Verification items for the finished model (mm, model axes). A direction names the side the tool comes from. Round coordinates to 2 decimals unless told otherwise and drop trailing zeros. Order: outer loops, then holes, each group sorted by start corner. A loop starts at its lowest first (then second) coordinate and runs counter-clockwise, first axis right, second up. Notation, with made-up numbers: (21.5, 54.25) -> (40.5, 54.25) arc R16 ccw to (40.5, 77.25) -> close; hole circle Ø3 at (6.5, 11.5). An arc over 180 degrees is marked (long way). Write item = value, one per line. Start each with the question number.
from build123d import *

# Parameters (mm, degrees)
SKETCH_1_W      = 80
SKETCH_1_H      = 59.5
EXTRUDE_1_DEPTH = 5
FILLET_1_R      = 1
EXTRUDE_2_DEPTH = 1
CHAMFER_1_SIZE  = 0.8
EXTRUDE_START   = -1
EXTRUDE_3_DEPTH = 1
CHAMFER_2_SIZE  = 0.8


with BuildPart() as part:
    # 草图1 → 凸台-拉伸1 (new body)
    with BuildSketch(Plane(origin=(0, 0, 0), x_dir=(1, 0, 0), z_dir=(0, 1, 0))):
        with Locations((59.287159713, -12.081031523)):
            Rectangle(SKETCH_1_W, SKETCH_1_H)
    extrude(amount=EXTRUDE_1_DEPTH)

    # 圆角1
    fillet_1_edges = [part.edges().sort_by_distance(p)[0] for p in [
        (59.287159713, 5, -17.668968477),
        (59.287159713, 0, -17.668968477),
        (59.287159713, 0, 41.831031523),
        (59.287159713, 5, 41.831031523),
    ]]
    fillet(fillet_1_edges, radius=FILLET_1_R)

    # 草图2 → 凸台-拉伸2 (add)
    with BuildSketch(Plane(origin=(99.287159713, 0, 0), x_dir=(0, 0, -1), z_dir=(1, 0, 0))):
        with BuildLine():
            Line((16.668968477, 5.5), (-40.831031523, 5.5))
            ThreePointArc((-40.831031523, 5.5), (-41.891691695, 5.060660172), (-42.331031523, 4))
            Line((-42.331031523, 4), (-42.331031523, 1))
            ThreePointArc((-42.331031523, 1), (-41.891691695, -0.060660172), (-40.831031523, -0.5))
            Line((-40.831031523, -0.5), (16.668968477, -0.5))
            ThreePointArc((16.668968477, -0.5), (17.729628648, -0.060660172), (18.168968477, 1))
            Line((18.168968477, 1), (18.168968477, 4))
            ThreePointArc((18.168968477, 4), (17.729628648, 5.060660172), (16.668968477, 5.5))
        make_face()
    extrude(amount=-EXTRUDE_2_DEPTH)

    # 倒角1
    chamfer_1_edges = [part.edges().sort_by_distance(p)[0] for p in [
        (99.287159713, 5.060660172, -17.729628648),
        (99.287159713, 5.5, 12.081031523),
        (99.287159713, 5.060660172, 41.891691695),
        (99.287159713, 2.5, 42.331031523),
        (99.287159713, -0.060660172, 41.891691695),
        (99.287159713, -0.5, 12.081031523),
        (99.287159713, -0.060660172, -17.729628648),
        (99.287159713, 2.5, -18.168968477),
    ]]
    chamfer(chamfer_1_edges, length=CHAMFER_1_SIZE)

    # 草图3 → 凸台-拉伸3 (add)
    with BuildSketch(Plane.ZY.offset(-19.287159713).offset(EXTRUDE_START)):
        with BuildLine():
            Line((40.831031523, 5.5), (-16.668968477, 5.5))
            ThreePointArc((-16.668968477, 5.5), (-17.729628648, 5.060660172), (-18.168968477, 4))
            Line((-18.168968477, 4), (-18.168968477, 1))
            ThreePointArc((-18.168968477, 1), (-17.729628648, -0.060660172), (-16.668968477, -0.5))
            Line((-16.668968477, -0.5), (40.831031523, -0.5))
            ThreePointArc((40.831031523, -0.5), (41.891691695, -0.060660172), (42.331031523, 1))
            Line((42.331031523, 1), (42.331031523, 4))
            ThreePointArc((42.331031523, 4), (41.891691695, 5.060660172), (40.831031523, 5.5))
        make_face()
    extrude(amount=EXTRUDE_3_DEPTH)

    # 倒角2
    chamfer_2_edges = [part.edges().sort_by_distance(p)[0] for p in [
        (19.287159713, 5.060660172, 41.891691695),
        (19.287159713, 5.5, 12.081031523),
        (19.287159713, 5.060660172, -17.729628648),
        (19.287159713, 2.5, -18.168968477),
        (19.287159713, -0.060660172, -17.729628648),
        (19.287159713, -0.5, 12.081031523),
        (19.287159713, -0.060660172, 41.891691695),
        (19.287159713, 2.5, 42.331031523),
    ]]
    chamfer(chamfer_2_edges, length=CHAMFER_2_SIZE)


solid = part.part
(1) Scan lines: line 1 along Y through (x, z) = (87.5, 34.5); line 2 along Z through (x, y) = (77.5, 3.75); line 3 along Z through (x, y) = (32, 4.75). Record each from-to range of solid material in increasing order. Write a range as from..to.
(2) Draft check along X on faces 1 (the flat face through (99.287, 3, 12)), 2 (the flat face through (59, 2, 41.831)), 3 (the flat face through (59, 0, 12)), 4 (the flat face through (19.287, 3, 12)). Enter one of: +X half, -X half, draft (parallel to the pull), parting line (faces both ways), or undercut.
(3) Depth check by flat-ended pin: pin 1 (8 mm diameter, centred on x = 90.5, z = -4.5, fed in from -Y); pin 2 (5 mm diameter, centred on x = 54, z = 5.5, fed in from +Y); pin 3 (3.5 mm diameter, centred on x = 71, y = 2.5, fed in from -Z). Enter the tip coordinate at first touch or a pass-through.
(4) Cross-section at B-B (z = -4). Enter the section's corners in (x, y).
(5) Cross-section at A-A (x = 69). Enter the section's corners in (y, z), and give its area (3 significant figures).
(6) Set-up check for faces 5 (the flat face through (59, 2, -17.669)), 6 (the flat face through (59, 5, 12)): record each of +Z, -Z, +X, -X, +Y, -Y from which the full face is reachable in a straight line by a thin tool's end or side.
Outcome:
q1.line_1 = 0..5
q1.line_2 = -17.67..41.83
q1.line_3 = -17.33..41.49
q2.face_1 = +X half
q2.face_2 = undercut
q2.face_3 = undercut
q2.face_4 = -X half
q3.pin_1 = 0
q3.pin_2 = 5
q3.pin_3 = -17.67
q4.outline = (19.29, 0.3) -> (20.09, -0.5) -> (20.29, -0.5) -> (20.29, 0) -> (98.29, 0) -> (98.29, -0.5) -> (98.49, -0.5) -> (99.29, 0.3) -> (99.29, 4.7) -> (98.49, 5.5) -> (98.29, 5.5) -> (98.29, 5) -> (20.29, 5) -> (20.29, 5.5) -> (20.09, 5.5) -> (19.29, 4.7) -> close
q5.outline = (0, -16.67) arc R1 ccw to (1, -17.67) -> (4, -17.67) arc R1 ccw to (5, -16.67) -> (5, 40.83) arc R1 ccw to (4, 41.83) -> (1, 41.83) arc R1 ccw to (0, 40.83) -> close
q5.area = 297 mm^2
q6.face_5 = -Z, +Y, -Y
q6.face_6 = +Z, -Z, +Y
